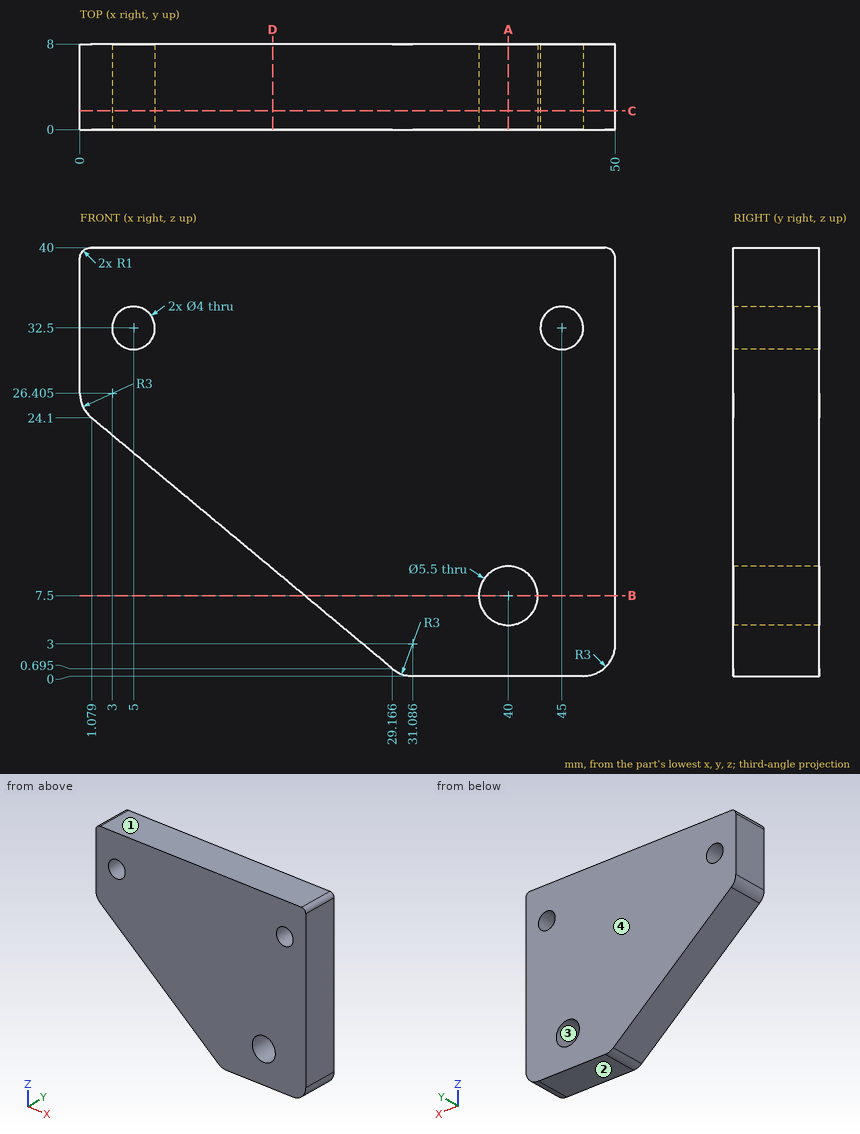
The figure shows three views and two pictorial views of one solid part (mm, origin at its lowest corner). Answer the questions. Give positions to 0.01 mm unless a question says otherwise; leave off trailing zeros. Order: outer loops, then holes, each group sorted by start corner. A loop starts at its lowest first (then second) coordinate and runs counter-clockwise, first axis right, second up. Notation, with made-up numbers: M -17,48 L 32,48 A19 ccw 32,69 Z; hole C 62,62 d5. An arc over 180 degrees is marked long. Return JSON: item names as keys, results as strings.
Q1. Find section A-A, the plane x = 40. Write down the section's boundary in (y, z).
Answer below:
{"outline": "M 0,0 L 8,0 L 8,4.75 L 0,4.75 Z; M 0,10.25 L 8,10.25 L 8,40 L 0,40 Z"}
Q2. Each of these flat-tipped pins is pushed along its axis until it touches: pin 1 (2 mm diameter, centred on x = 15, y = 3.5, fed in from -Z); pin 2 (3 mm diameter, centred on x = 7, z = 17, fed in from +Y); pin 3 (3 mm diameter, centred on y = 2.5, z = 17.5, fed in from -X). Where does it stop, or does it pass through?
Answer below:
{"pin 1": "stops at z = 11.67", "pin 2": "passes through", "pin 3": "stops at x = 7.2"}
Q3. Find section C-C, the plane y = 1.75. State how many separate pieces and enclosed holes the cut face has, and give its area (3 significant figures).
Answer below:
{"separate pieces": "1", "enclosed holes": "3", "area": "1,570 mm^2"}
Q4. Find section B-B, the plane z = 7.5. Write down the section's boundary in (x, y), and give its area (3 significant figures).
Answer below:
{"outline": "M 21,0 L 37.25,0 L 37.25,8 L 21,8 Z; M 42.75,0 L 50,0 L 50,8 L 42.75,8 Z", "area": "188 mm^2"}
Q5. Find section D-D, the plane x = 18. Write down the section's boundary in (y, z).
Answer below:
{"outline": "M 0,10 L 8,10 L 8,40 L 0,40 Z"}
Q6. Find the intervals of material crossed by line 1 along Z through (x, y) = (40, 3); line 2 along X through (y, z) = (5, 32.5); line 3 along Z through (x, y) = (45, 2.75), in increasing order. Write a range as [from, to].
Answer below:
{"line 1": "z = [0, 4.75], [10.25, 40]", "line 2": "x = [0, 3], [7, 43], [47, 50]", "line 3": "z = [0, 30.5], [34.5, 40]"}
Q7. The mould has two halves that part along Z. Classify the marked faces 1, 2, 3 and 4: pulls with the +Z half, pulls with the -Z half, needs draft (parallel to the pull), parting line crosses it, or undercut.
Answer below:
{"face 1": "pulls with the +Z half", "face 2": "pulls with the -Z half", "face 3": "undercut", "face 4": "needs draft"}
